Here's how the part is built. I have some questions about the finished solid (model axes, mm). Give positions to 0.01 mm unless a question says otherwise; leave off trailing zeros. Write each loop counter-clockwise with the first axis right and the second up, starting at its lowest first coordinate (ties: lowest second). Pieces come first, ordered by that corner, then holes. Notation, with made-up numbers: (89.25, -1) -> (115.25, -1) arc R37 cw to (115.25, 36) -> close; hole circle Ø11 at (-26.75, 35). An arc over 180 degrees is marked (long way). Use one line per item in the form item = value.
```python
from build123d import *

# Parameters (mm, degrees)
F1_DEPTH = 2
F2_R     = 1.5
F3_DEPTH = 2
F4_R     = 1
F5_DEPTH = 2
F6_R     = 0.512692
F7_DEPTH = 1
F8_R     = 0.507408
F9_DEPTH = 1


with BuildPart() as f1:
    # F0 (on Right) → F1 (new body)
    with BuildSketch(Plane.YZ):
        with BuildLine():
            ThreePointArc((2.152867, -2.751681), (1.644867, -2.243681), (1.136867, -2.751681))
            ThreePointArc((1.136867, -2.751681), (1.644867, -3.259681), (2.152867, -2.751681))
        make_face()
        with BuildLine():
            ThreePointArc((4.184458, -1.435063), (4.035669, -1.075853), (3.676458, -0.927063))
            ThreePointArc((3.676458, -0.927063), (3.317248, -1.794273), (4.184458, -1.435063))
        make_face()
        Polygon((3.676458, 0), (0, 0), (0, -2.751681), (0, -4), (160.02, -2), (160.02, 0), align=None)
        with BuildLine():
            ThreePointArc((2.152867, -2.751681), (1.644867, -3.259681), (1.136867, -2.751681))
            ThreePointArc((1.136867, -2.751681), (1.644867, -2.243681), (2.152867, -2.751681))
        make_face(mode=Mode.SUBTRACT)
        with BuildLine():
            ThreePointArc((4.184458, -1.435063), (3.317248, -1.794273), (3.676458, -0.927063))
            ThreePointArc((3.676458, -0.927063), (4.035669, -1.075853), (4.184458, -1.435063))
        make_face(mode=Mode.SUBTRACT)
    extrude(amount=F1_DEPTH)

    # F2 (on face) → F3 (join)
    with BuildSketch(Plane(origin=(0, 160.02, 0), x_dir=(-1, 0, 0), z_dir=(0, 1, 0))):
        with BuildLine():
            ThreePointArc((0, -0.091288), (1.09165, 0.830694), (1.5, 2.2))
            ThreePointArc((1.5, 2.2), (-2.369306, 4.29165), (-2, -0.091288))
            Line((-2, -0.091288), (-2, 0))
            Line((-2, 0), (0, 0))
            Line((0, 0), (0, -0.091288))
        make_face()
        with Locations((-1, 2.2)):
            Circle(F2_R, mode=Mode.SUBTRACT)
    extrude(amount=-F3_DEPTH)

    # F4 (on face) → F5 (join)
    with BuildSketch(Plane.XZ):
        with BuildLine():
            Line((2, 0), (2, 0.763859))
            ThreePointArc((2, 0.763859), (1, 3.95), (0, 0.763859))
            Line((0, 0.763859), (0, 0))
            Line((0, 0), (2, 0))
        make_face()
        with Locations((1, 2.2)):
            Circle(F4_R, mode=Mode.SUBTRACT)
    extrude(amount=-F5_DEPTH)

    # F6 (on face) → F7 (join)
    with BuildSketch(Plane.YZ.offset(2)):
        Polygon((5.441279, 0), (2.750172, 0), (2.750172, -3.965627), (5.441279, -3.931993), align=None)
        with Locations((3.676458, -1.435063)):
            Circle(F6_R, mode=Mode.SUBTRACT)
    extrude(amount=F7_DEPTH)

    # F8 (on face) → F9 (join)
    with BuildSketch(Plane(origin=(0, 0, 0), x_dir=(0, -1, 0), z_dir=(-1, 0, 0))):
        Polygon((-2.654617, 0), (-5.185953, 0), (-5.186794, -3.935173), (-2.654617, -3.966821), align=None)
        with Locations((-3.676458, -1.435063)):
            Circle(F8_R, mode=Mode.SUBTRACT)
    extrude(amount=F9_DEPTH)


solid = f1.part
```
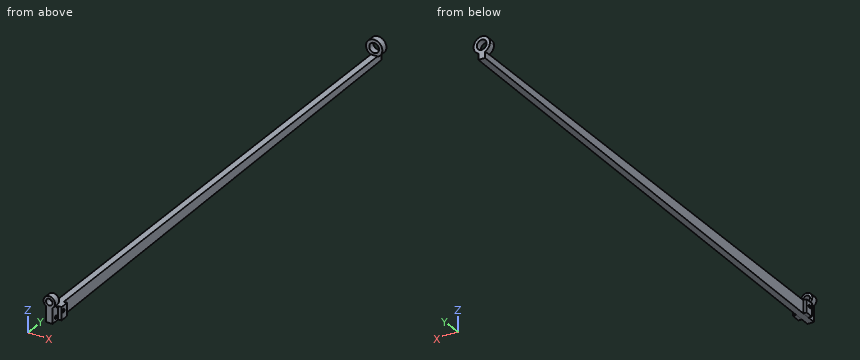
Q1. I want a section at A-A, the plane x = 0.9. Write out the boundary of the cut face in (y, z), and give its area (3 significant figures).
Result set:
outline = (0, -4) -> (160.02, -2) -> (160.02, 0.7) -> (158.02, 0.7) -> (158.02, 0) -> (2, 0) -> (2, 1.21) -> (0, 1.21) -> close; (0, 3.19) -> (2, 3.19) -> (2, 3.95) -> (0, 3.95) -> close; (158.02, 3.7) -> (160.02, 3.7) -> (160.02, 4.7) -> (158.02, 4.7) -> close; hole circle Ø1.02 at (1.64, -2.75); hole circle Ø1.02 at (3.68, -1.44)
area = 486 mm2
Q2. I want a section at B-B, the plane y = 149. Write out the boundary of the cut face in (x, z), and give its area (3 significant figures).
Result set:
outline = (0, -2.14) -> (2, -2.14) -> (2, 0) -> (0, 0) -> close
area = 4.28 mm2
Q3. If I drill on line 1 along Y through (x, z) = (2.2, 1.25); line 2 along X through (y, z) = (81.5, -1.75); line 3 along Z through (x, y) = (1, 159.4), over which ranges is the centre line in solid material (lowest first)? Write a range as from..to.
Result set:
line_1 = 0..2, 158.02..160.02
line_2 = 0..2
line_3 = -2.01..0.7, 3.7..4.7
Q4. Will these pins go through, and if not, where does the flat tip stop? pin 1 Ø0.8 at (x, z) = (-0.5, -2.5) entering from -Y; pin 2 Ø4 at (y, z) = (4, -1) entering from -X; pin 3 Ø2 at (y, z) = (52.5, -3) entering from -X; pin 4 Ø1.5 at (y, z) = (45, 2) entering from -X (3 decimals).
Result set:
pin_1 = 2.65
pin_2 = -1
pin_3 = 0
pin_4 = through
Q5. I want a section at C-C, the plane y = 28.5. Write out the boundary of the cut face in (x, z).
Result set:
outline = (0, -3.64) -> (2, -3.64) -> (2, 0) -> (0, 0) -> close
